Read the model definition and answer for the solid it produces. Units are mm, in the model's axes. Face numbers are marked on the shaded views. A direction names the side the tool comes from. Coordinates: 2 decimals unless noted, no trailing zeros. Order: outer loops, then holes, each group sorted by start corner. A loop starts at its lowest first (then second) coordinate and runs counter-clockwise, first axis right, second up.
Solid Edge part; units mm, degrees
sketch "Sketch1" plane through (0, 0, 0) normal (0, -1, 0) x (1, 0, 0)
  line L0 (-40, -7.5) -> (40, -7.5)
  line L1 (40, -7.5) -> (40, 7.5)
  line L2 (40, 7.5) -> (-40, 7.5)
  line L3 (-40, 7.5) -> (-40, -7.5)
  dimension "D1" = 40
  dimension "D2" = 40
extrude "Protrusion1" add sketch "Sketch1" along normal mid plane 35
chamfer "Chamfer_1" distance 2 angle 45 8 edges at (40, 0, 7.5) (40, 17.5, 0) (40, 0, -7.5) (0, 17.5, 7.5) (0, 17.5, -7.5) (-40, 0, -7.5) (-40, 0, 7.5) (-40, 17.5, 0)
hole "Hole_1" at (-20, 0, 7.5) direction (0, 0, -1) diameter 16 end up to next start chamfer 0.6 start chamfer angle 30 end chamfer 0.6 end chamfer angle 30
hole "Hole_2" at (30, 0, 7.5) direction (0, 0, -1) diameter 9 end up to next start chamfer 0.6 start chamfer angle 45 end chamfer 0.6 end chamfer angle 45
sketch "Sketch2" plane through (0, -17.5, 0) normal (0, -1, 0) x (1, 0, 0)
  line L0 (-38, 7.5) -> (-38, -7.5)
  line L1 (-38, -7.5) -> (-50, -7.5)
  line L2 (-50, -7.5) -> (-50, 7.5)
  line L3 (-50, 7.5) -> (-38, 7.5)
  line L4 (38, 7.5) -> (38, -7.5)
  line L5 (38, -7.5) -> (50, -7.5)
  line L6 (50, -7.5) -> (50, 7.5)
  line L7 (50, 7.5) -> (38, 7.5)
extrude "ExtrudedProtrusion_2" add sketch "Sketch2" against normal blind 6
hole "Hole_3" at (-45, -17.5, 0) direction (0, 1, 0) diameter 2.85 depth 30 tip angle 118 start chamfer 0.6 start chamfer angle 30 end chamfer 0.6 end chamfer angle 30
hole "Hole1" at (45, -17.5, 0) direction (0, 1, 0) diameter 2.85 depth 30 tip angle 118 start chamfer 0.6 start chamfer angle 30 end chamfer 0.6 end chamfer angle 30
hole "Hole2" at (0, -17.5, 0) direction (0, 1, 0) diameter 2.85 depth 30 tip angle 118 start chamfer 0.6 start chamfer angle 30 end chamfer 0.6 end chamfer angle 30
hole "Hole_5" at (-31, 0, 7.5) direction (0, 0, -1) diameter 2.85 depth 30 tip angle 118 start chamfer 0.6 start chamfer angle 30 end chamfer 0.6 end chamfer angle 30
pattern_circular "Pattern2" count 4 over 360 about axis through (-20, 0, 6.4608) along (0, 0, 1) of "Hole_5"
properties material "Polyethylene, low density"
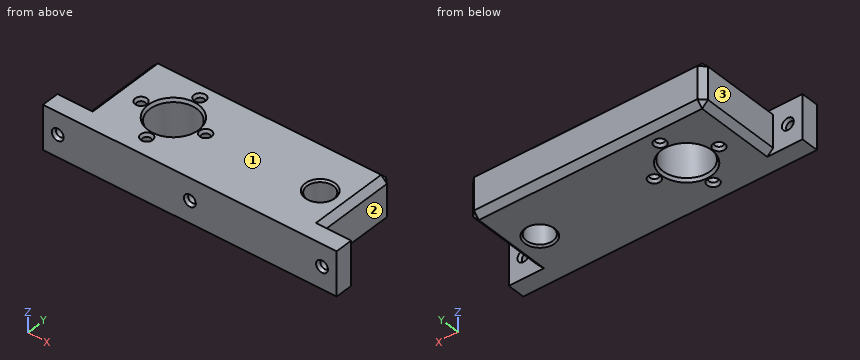
1) A cutting plane is placed at C-C, the plane y = 0. State how many separate pieces and enclosed holes the cut face has, and give its area (3 significant figures).
A:
separate pieces: 5
enclosed holes: 1
area: 721 mm2
2) Which of the six approach directions +Z, -Z, +X, -X, +Y, -Y give full straight-line access (tool end or side, diameter ignored) to the marked faces 1, 2 and 3?
A:
face 1: +Z, +X, -X, +Y, -Y
face 2: +Z, -Z, +X, +Y
face 3: +Z, -Z, -X, +Y
3) Flat-ended cylindrical pins translate along their axes: pin 1 Ø3.5 at (y, z) = (-1.5, -1) entering from -X; pin 2 Ø3.5 at (x, z) = (45, 3) entering from +Y; pin 3 Ø4 at (y, z) = (-2, -0.5) entering from +X. Find the tip coordinate at first contact, or state that the pin passes through.
A:
pin 1: stops at x = -40
pin 2: stops at y = -11.5
pin 3: stops at x = 40
4) A cutting plane is placed at A-A, the plane x = 30. Determine the outline of the cut face in (y, z), and give its area (3 significant figures).
A:
outline: (-17.5, -7.5) - (-5.1, -7.5) - (-4.5, -6.9) - (-4.5, 6.9) - (-5.1, 7.5) - (-17.5, 7.5) - close; (4.5, -6.9) - (5.1, -7.5) - (15.5, -7.5) - (17.5, -5.5) - (17.5, 5.5) - (15.5, 7.5) - (5.1, 7.5) - (4.5, 6.9) - close
area: 385 mm2
5) Straight lines are drawn through the part: line 1 (Y direction, x = -20, z = 1.25) (3 decimals); line 2 (X direction, y = 0, z = 1.5) (3 decimals); line 3 (X direction, y = -11, z = 0.75) (3 decimals). For each, find the intervals that lie inside material, in ascending order.
A:
line 1: y = -17.5 to -12.425, -9.575 to -8, 8 to 9.575, 12.425 to 17.5
line 2: x = -40 to -32.425, -29.575 to -28, -12 to -10.425, -7.575 to 25.5, 34.5 to 40
line 3: x = -40 to -21.425, -18.575 to -1.212, 1.212 to 40
6) A cutting plane is placed at B-B, the plane z = -3.5. Determine the outline of the cut face in (x, y) (3 decimals).
A:
outline: (-50, -17.5) - (50, -17.5) - (50, -11.5) - (40, -11.5) - (40, 15.5) - (38, 17.5) - (-38, 17.5) - (-40, 15.5) - (-40, -11.5) - (-50, -11.5) - close; hole circle Ø2.85 at (-31, 0); hole circle Ø16 at (-20, 0); hole circle Ø2.85 at (-20, -11); hole circle Ø2.85 at (-20, 11); hole circle Ø2.85 at (-9, 0); hole circle Ø9 at (30, 0)
